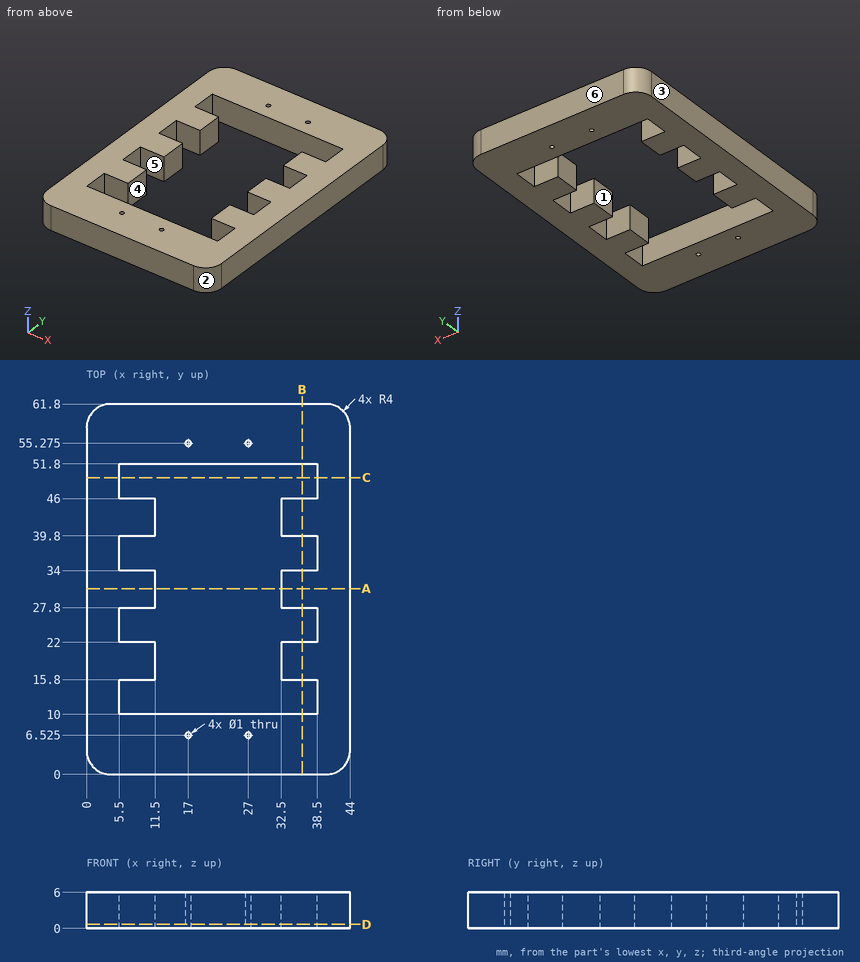
Study the drawing (mm; zero at the part's minimum x, y, z) and answer. A direction names the side the tool comes from. Round coordinates to 2 decimals unless told otherwise and drop trailing zeros. Write each loop counter-clockwise with the first axis right and the second up, starting at its lowest first coordinate (ties: lowest second). Pieces come first, ordered by that corner, then holes.
1) A cutting plane is placed at C-C on y = 49.5. Determine the outline of the cut face in (x, z), and give its area (3 significant figures).
2) Which of the six approach directions +Z, -Z, +X, -X, +Y, -Y give full straight-line access (tool end or side, diameter ignored) to the marked faces 5 and 6?
3) A cutting plane is placed at D-D on z = 0.65. Give the number of separate pieces and of enclosed holes in the cut face, and give its area (3 significant figures).
4) A flat-ended cylindrical pin translates along its axis: P1, Ø3, axis at x = 29.5, y = 31, coming from the +Z side. Find the tip coordinate at first contact, or state that the pin passes through.
5) A cutting plane is placed at A-A on y = 31. Determine the outline of the cut face in (x, z).
6) A cutting plane is placed at B-B on x = 36. Determine the outline of the cut face in (y, z).
7) Consider probe 1 along Y at (x, z) = (17, 2.1) (3 decimals); probe 2 along Y at (x, z) = (33, 3.9); probe 3 along Y at (x, z) = (29.5, 4). Determine where each line is inside the solid, lowest interval first.
8) Determine the mould class of the marked faces 1, 2, 3 and 4 for opening direction Y: pulls with the +Y half, pulls with the -Y half, needs draft (parallel to the pull), parting line crosses it, or undercut.
Entries:
1. outline: (0, 0) - (5.5, 0) - (5.5, 6) - (0, 6) - close; (38.5, 0) - (44, 0) - (44, 6) - (38.5, 6) - close
1. area: 66.0 mm2
2. face 5: +Z, -Z
2. face 6: +Z, -Z, +X, -X, +Y
3. separate pieces: 1
3. enclosed holes: 5
3. area: 1,550 mm2
4. P1: passes through
5. outline: (0, 0) - (11.5, 0) - (11.5, 6) - (0, 6) - close; (32.5, 0) - (44, 0) - (44, 6) - (32.5, 6) - close
6. outline: (0, 0) - (10, 0) - (10, 6) - (0, 6) - close; (15.8, 0) - (22, 0) - (22, 6) - (15.8, 6) - close; (27.8, 0) - (34, 0) - (34, 6) - (27.8, 6) - close; (39.8, 0) - (46, 0) - (46, 6) - (39.8, 6) - close; (51.8, 0) - (61.8, 0) - (61.8, 6) - (51.8, 6) - close
7. probe 1: y = 0 to 6.025, 7.025 to 10, 51.8 to 54.775, 55.775 to 61.8
7. probe 2: y = 0 to 10, 15.8 to 22, 27.8 to 34, 39.8 to 46, 51.8 to 61.8
7. probe 3: y = 0 to 10, 51.8 to 61.8
8. face 1: undercut
8. face 2: pulls with the -Y half
8. face 3: needs draft
8. face 4: undercut
